Here's how the part is built. I have some questions about the finished solid (model axes, mm). A direction names the side the tool comes from. Coordinates: 2 decimals unless noted, no trailing zeros. Write each loop counter-clockwise with the first axis right and the second up, starting at its lowest first coordinate (ties: lowest second). Pieces come first, ordered by that corner, then holes. Notation, with made-up numbers: (-5, 0.5) -> (46, 0.5) arc R24 ccw to (46, 17.5) -> close; hole circle Ø4 at (-7, 52). An arc over 180 degrees is marked (long way). Answer in a Markdown table with one row per item. Add a question column.
from build123d import *

# Parameters (mm, degrees)
SKETCH1_R           = 6
BOSS_EXTRUDE1_DEPTH = 21
SKETCH2_R           = 3.4
CUT_EXTRUDE1_DEPTH  = 23.649503306
CUT_EXTRUDE2_DEPTH  = 5
CHAMFER1_SIZE       = 0.5


with BuildPart() as part:
    # Sketch1 → Boss-Extrude1 (new body)
    with BuildSketch(Plane(origin=(0, 0, 0), x_dir=(1, 0, 0), z_dir=(0, 1, 0))):
        with Locations(Location((0, 0, 0), (0, 0, 270))):
            Circle(SKETCH1_R)
    extrude(amount=-BOSS_EXTRUDE1_DEPTH)

    # Sketch2 → Cut-Extrude1 (cut, through all)
    with BuildSketch(Plane(origin=(0, 0, 0), x_dir=(1, 0, 0), z_dir=(0, 1, 0))):
        with Locations(Location((0, 0, 0), (0, 0, 270))):
            Circle(SKETCH2_R)
    extrude(amount=-CUT_EXTRUDE1_DEPTH, mode=Mode.SUBTRACT)

    # Sketch3 → Cut-Extrude2 (cut)
    with BuildSketch(Plane(origin=(0, 0, 0), x_dir=(1, 0, 0), z_dir=(0, 1, 0))):
        Polygon((4.618802154, 0), (2.309401077, 4), (-2.309401077, 4), (-4.618802154, 0), (-2.309401077, -4), (2.309401077, -4), align=None)
    extrude(amount=-CUT_EXTRUDE2_DEPTH, mode=Mode.SUBTRACT)

    # Chamfer1
    chamfer1_edges = [part.edges().sort_by_distance(p)[0] for p in [
        (0, 0, -6),
        (0, -21, -6),
    ]]
    chamfer(chamfer1_edges, length=CHAMFER1_SIZE)


solid = part.part
Q1. I need wall thicknesses on line 1 (X direction, y = -8.25, z = 0); line 2 (X direction, y = -5.75, z = -2.75); line 3 (Z direction, x = 2.5, y = -1.25). Which ranges of each line are inside material? Lowest first, please. Write a range as [from, to].
Q2. I'm going to push flat-ended pins straight in: P1, Ø6, axis at x = 4, z = 5, coming from the -Y side; P2, Ø1.5, axis at y = -13.5, z = 2, coming from the +X side. Where does each tip first touch, or does it pass through?
Q3. Imagine slicing it at B-B on y = -16.5. Please give me the cut outline in (x, z), plus the area to 3 significant figures.
Q4. If we mould it in two halves opening along Z, with no side actions, what happens to faces 3 (the flat face through (-3.448, -2.465, -2.028)), 4 (the cylindrical face through (1.802, -10.36, 5.723)), 5 (the flat face through (4, 0, -2))? For each: pulls with the +Z half, pulls with the -Z half, needs draft (parallel to the pull), parting line crosses it, or undercut.
Q5. Imagine slicing it at A-A on x = 0. Please give me the cut outline in (y, z), plus the area to 3 significant figures.
Q6. For faces 1 (the flat face through (0, -2, -4)), 2 (the flat face through (-2, -21, -3)), which set-ups out of +Z, -Z, +X, -X, +Y, -Y let a thin tool reach every point of the face, with its end or its side?
Result sheet:
| question | item | result |
|---|---|---|
| 1 | line 1 | x = [-6, -3.4], [3.4, 6] |
| 1 | line 2 | x = [-5.33, -2], [2, 5.33] |
| 1 | line 3 | z = [-5.45, -3.67], [3.67, 5.45] |
| 2 | P1 | stops at y = -21 |
| 2 | P2 | stops at x = 5.87 |
| 3 | outline | circle Ø12 at (0, 0); hole circle Ø6.8 at (0, 0) |
| 3 | area | 76.8 mm^2 |
| 4 | face 3 | undercut |
| 4 | face 4 | parting line crosses it |
| 4 | face 5 | needs draft |
| 5 | outline | (-21, -5.5) -> (-20.5, -6) -> (-0.5, -6) -> (0, -5.5) -> (0, -4) -> (-5, -4) -> (-5, -3.4) -> (-21, -3.4) -> close; (-21, 3.4) -> (-5, 3.4) -> (-5, 4) -> (0, 4) -> (0, 5.5) -> (-0.5, 6) -> (-20.5, 6) -> (-21, 5.5) -> close |
| 5 | area | 103 mm^2 |
| 6 | face 1 | +Y |
| 6 | face 2 | +Z, -Z, +X, -X, -Y |
